Source: CAD feature listing. Evaluate the final solid. Frame: model axes, mm. Face numbers are marked on the shaded views. A direction names the side the tool comes from. Give positions to 0.01 mm unless a question says otherwise; leave off trailing zeros. Write each loop counter-clockwise with the first axis right and the second up, starting at its lowest first coordinate (ties: lowest second). Pieces come first, ordered by that corner, then holes.
```python
from build123d import *

# Parameters (mm, degrees)
SKETCH1_W                      = 150
SKETCH1_H                      = 150
BOSS_EXTRUDE1_DEPTH            = 20
SKETCH2_W                      = 80
SKETCH2_H                      = 80
BOSS_EXTRUDE2_DEPTH            = 40
SKETCH3_W                      = 150
SKETCH3_H                      = 150
BOSS_EXTRUDE3_DEPTH            = 30
HOLE2_D                        = 27
HOLE2_CBORE_D                  = 60
HOLE2_CBORE_DEPTH              = 10
M16_START                      = 60
M16_TAPPED_HOLE1_OUTLINE_R     = 7
M16_TAPPED_HOLE1_DEPTH         = 30
F_10_0_10_DIAMETER_HOLE1_D     = 10
F_10_0_10_DIAMETER_HOLE1_DEPTH = 14.995696905
F_10_0_10_DIAMETER_HOLE1_TIP   = 3.004303095
FILLET1_R                      = 3
CHAMFER1_SIZE                  = 2


# Read off the part's stored shape, not the designer's step: M16 Tapped Hole1
with BuildPart() as part:
    # Sketch1 → Boss-Extrude1 (new body)
    with BuildSketch(Plane(origin=(0, 0, 0), x_dir=(1, 0, 0), z_dir=(0, 1, 0))):
        Rectangle(SKETCH1_W, SKETCH1_H)
    extrude(amount=BOSS_EXTRUDE1_DEPTH)

    # Sketch2 → Boss-Extrude2 (add)
    with BuildSketch(Plane(origin=(0, 20, 0), x_dir=(1, 0, 0), z_dir=(0, 1, 0))):
        Rectangle(SKETCH2_W, SKETCH2_H)
    extrude(amount=BOSS_EXTRUDE2_DEPTH)

    # Sketch3 → Boss-Extrude3 (add)
    with BuildSketch(Plane(origin=(0, 60, 0), x_dir=(1, 0, 0), z_dir=(0, 1, 0))):
        Rectangle(SKETCH3_W, SKETCH3_H)
    extrude(amount=BOSS_EXTRUDE3_DEPTH)

    # Hole2 (through all)
    with Locations(Plane(origin=(0, 0, 0), x_dir=(0, 0, -1), z_dir=(0, -1, 0))):
        with Locations((0, 0)):
            CounterBoreHole(HOLE2_D / 2, HOLE2_CBORE_D / 2, HOLE2_CBORE_DEPTH)

    # M16 Tapped Hole1 outline → M16 Tapped Hole1 (cut)
    with BuildSketch(Plane(origin=(0, 0, 0), x_dir=(1, 0, 0), z_dir=(0, 1, 0)).offset(M16_START)):
        with Locations((-60, 0)):
            Circle(M16_TAPPED_HOLE1_OUTLINE_R)
        with Locations((0, -60)):
            Circle(M16_TAPPED_HOLE1_OUTLINE_R)
        with Locations((60, 0)):
            Circle(M16_TAPPED_HOLE1_OUTLINE_R)
        with Locations((0, 60)):
            Circle(M16_TAPPED_HOLE1_OUTLINE_R)
        with Locations((60, -60)):
            Circle(M16_TAPPED_HOLE1_OUTLINE_R)
        with Locations((-60, 60)):
            Circle(M16_TAPPED_HOLE1_OUTLINE_R)
        with Locations((-60, -60)):
            Circle(M16_TAPPED_HOLE1_OUTLINE_R)
        with Locations((60, 60)):
            Circle(M16_TAPPED_HOLE1_OUTLINE_R)
    extrude(amount=M16_TAPPED_HOLE1_DEPTH, mode=Mode.SUBTRACT)

    # Ø10.0 (10) Diameter Hole1
    with Locations(Plane(origin=(0, 0, 0), x_dir=(-1, 0, 0), z_dir=(0, -1, 0))):
        with Locations((0, 0), (0, -60), (60, 0), (-60, 0), (0, 60)):
            Hole(F_10_0_10_DIAMETER_HOLE1_D / 2, depth=F_10_0_10_DIAMETER_HOLE1_DEPTH)
            with Locations((0, 0, -(F_10_0_10_DIAMETER_HOLE1_DEPTH + F_10_0_10_DIAMETER_HOLE1_TIP / 2))):  # 118° drill point
                Cone(0, F_10_0_10_DIAMETER_HOLE1_D / 2, F_10_0_10_DIAMETER_HOLE1_TIP, mode=Mode.SUBTRACT)

    # Fillet1
    fillet1_edges = [part.edges().sort_by_distance(p)[0] for p in [
        (40, 20, 0),
        (0, 20, -40),
        (-40, 20, 0),
        (0, 20, 40),
    ]]
    fillet(fillet1_edges, radius=FILLET1_R)

    # Chamfer1
    chamfer1_edges = [part.edges().sort_by_distance(p)[0] for p in [
        (0, 0, 30),
    ]]
    chamfer(chamfer1_edges, length=CHAMFER1_SIZE)


solid = part.part
```
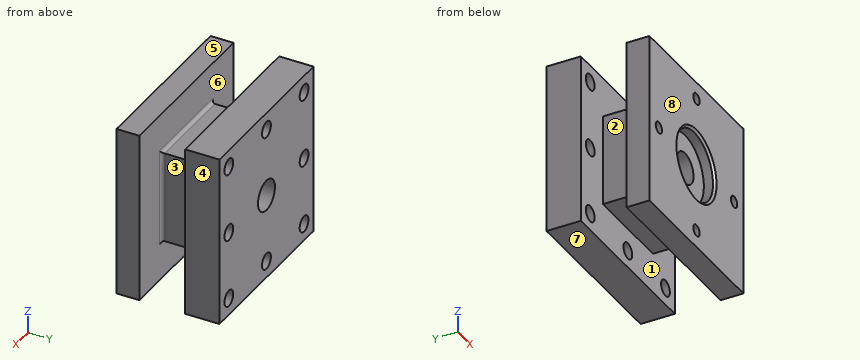
1. Access query for the marked faces 1, 2, 3, 4 and 5. Directions: +Z, -Z, +X, -X, +Y, -Y. A direction counts if a zero-diameter tool reaches every point of the face in a straight line with its end or side. Return the directions, or none.
2. Line query: probe 1 along X at (y, z) = (79, 60); probe 2 along Y at (x, z) = (23, -65.5). Output: solid intervals per line, ascending.
3. Section query D-D (x = 63). Give the number of separate pieces and of enclosed holes in the cut face, plus the area to 3 significant figures.
4. Pin query (flat end, axial travel): P1, Ø11, axis at x = -20, y = 33, coming from the -Z side; P2, Ø8.5, axis at x = 60, z = -60, coming from the -Y side; P3, Ø3, axis at y = 22.5, z = 37, coming from the -X side; P4, Ø8.5, axis at x = 60, z = 60, coming from the +Y side. Return the tip coordinate at first contact, or that it passes through.
5. Section query A-A (z = -50). Return loops of the section in (x, y), plus the area to 3 significant figures.
6. Pull-direction query (Y, two-part tool) for the marked faces 6, 7 and 8; classes: pulls with the +Y half, pulls with the -Y half, needs draft (parallel to the pull), parting line crosses it, or undercut.
7. Section query B-B (y = 44). Return loops of the section in (x, z), plus the area to 3 significant figures.
8. Section query C-C (x = -35.5). Return loops of the section in (y, z), plus the area to 3 significant figures.
The answers:
1. face 1: none
1. face 2: +Z, -Z, -X
1. face 3: +Z, -Z, +X
1. face 4: +Z, -Z, +X, +Y, -Y
1. face 5: +Z, +X, -X, +Y, -Y
2. probe 1: x = -75 to -67, -53 to -7, 7 to 53, 67 to 75
2. probe 2: y = 0 to 20, 60 to 90
3. separate pieces: 5
3. enclosed holes: 0
3. area: 6,240 mm2
4. P1: stops at z = -40
4. P2: stops at y = 0
4. P3: stops at x = -40.76
4. P4: stops at y = 20
5. outline: (-75, 0) - (75, 0) - (75, 20) - (-75, 20) - close; (-75, 60) - (75, 60) - (75, 90) - (-75, 90) - close
5. area: 7,500 mm2
6. face 6: undercut
6. face 7: needs draft
6. face 8: pulls with the -Y half
7. outline: (-40, -40) - (40, -40) - (40, 40) - (-40, 40) - close; hole circle Ø27 at (0, 0)
7. area: 5,830 mm2
8. outline: (0, -75) - (20, -75) - (20, -43) arc R3 cw to (23, -40) - (60, -40) - (60, -75) - (90, -75) - (90, 75) - (60, 75) - (60, 40) - (23, 40) arc R3 cw to (20, 43) - (20, 75) - (0, 75) - close
8. area: 10,700 mm2
